```python
from build123d import *

# Parameters (mm, degrees)
ESTRUSIONE_ESTRUSIONE1_DEPTH           = 20
FORO_SVASATO_PER_VITE_M4_1_D           = 4.5
FORO_SVASATO_PER_VITE_M4_1_DEPTH       = 30
FORO_SVASATO_PER_VITE_M4_1_CSINK_D     = 9.4
FORO_SVASATO_PER_VITE_M4_1_CSINK_ANGLE = 90
FORO_SVASATO_PER_VITE_M4_1_TIP         = 1.351936393


with BuildPart() as part:
    # Schizzo1 → Estrusione-Estrusione1 (new body)
    with BuildSketch(Plane.XY):
        with BuildLine():
            Line((-88.074783565, -50.85), (-79.414529527, -45.85))
            ThreePointArc((-79.414529527, -45.85), (-79.414529527, 45.85), (0, 91.7))
            Line((0, 91.7), (0, 101.7))
            ThreePointArc((0, 101.7), (-88.074783565, 50.85), (-88.074783565, -50.85))
        make_face()
        with BuildLine():
            Line((-77.906719865, -65.371499905), (-70.246275434, -58.943623808))
            ThreePointArc((-70.246275434, -58.943623808), (-75.116242461, -52.596959213), (-79.414529527, -45.85))
            Line((-79.414529527, -45.85), (-88.074783565, -50.85))
            ThreePointArc((-88.074783565, -50.85), (-83.307762904, -58.332723577), (-77.906719865, -65.371499905))
        make_face()
    extrude(amount=ESTRUSIONE_ESTRUSIONE1_DEPTH)

    # Foro svasato per Vite M4-1
    with Locations(Plane(origin=(-88.074783565, -50.85, 10), x_dir=(0.5, -0.866025403784, 0), z_dir=(-0.866025403784, -0.5, 0))):
        with Locations((0, 0)):
            CounterSinkHole(FORO_SVASATO_PER_VITE_M4_1_D / 2, FORO_SVASATO_PER_VITE_M4_1_CSINK_D / 2, depth=FORO_SVASATO_PER_VITE_M4_1_DEPTH, counter_sink_angle=FORO_SVASATO_PER_VITE_M4_1_CSINK_ANGLE)
            with Locations((0, 0, -(FORO_SVASATO_PER_VITE_M4_1_DEPTH + FORO_SVASATO_PER_VITE_M4_1_TIP / 2))):  # 118° drill point
                Cone(0, FORO_SVASATO_PER_VITE_M4_1_D / 2, FORO_SVASATO_PER_VITE_M4_1_TIP, mode=Mode.SUBTRACT)


solid = part.part
```
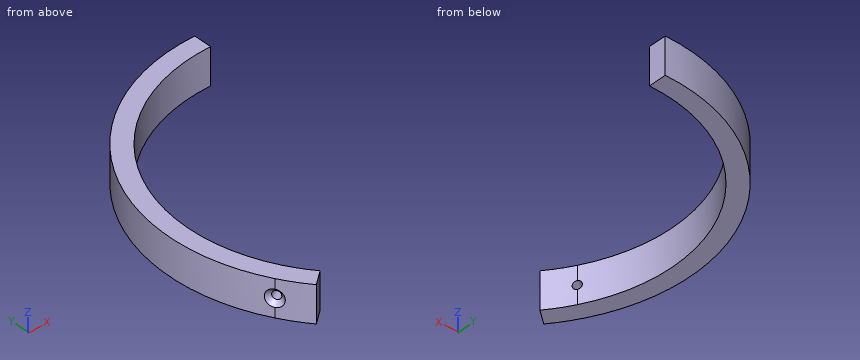
Geometry check sheet. Reference: the model listing, model coordinates, mm. Round coordinates to 2 decimals unless told otherwise and drop trailing zeros. Write each loop counter-clockwise with the first axis right and the second up, starting at its lowest first coordinate (ties: lowest second). Pieces come first, ordered by that corner, then holes. Notation, with made-up numbers: (40, -30) -> (64, -30) arc R23 cw to (64, 0) -> close; hole circle Ø8 at (68.25, -18.5). An arc over 180 degrees is marked (long way). Put each result on its own line as item: value.
1) Depth check by flat-ended pin: P1, Ø4, axis at y = 13, z = 4, coming from the -X side; P2, Ø3, axis at y = -26, z = 2.5, coming from the +X side; P3, Ø1, axis at x = -88, z = 11.5, coming from the -Y side. Enter the tip coordinate at first touch or a pass-through.
Recorded:
P1: stops at x = -101.1
P2: stops at x = -87.48
P3: stops at y = -48.02
2) Cross-section at B-B, the plane x = -29.5. Enter the section's corners in (y, z).
Recorded:
outline: (86.83, 0) -> (97.33, 0) -> (97.33, 20) -> (86.83, 20) -> close
3) Thickness scan on probe 1 along Y at (x, z) = (-83.5, 2.75); probe 2 along Y at (x, z) = (-83, 2.75); probe 3 along X at (y, z) = (-56, 9.5). Record the ranges inside material, lowest first. Write a range as from..to.
Recorded:
probe 1: y = -58.06..-37.9, 37.9..58.06
probe 2: y = -58.77..-38.99, 38.99..58.77
probe 3: x = -84.89..-72.61
4) Cross-section at C-C, the plane y = 19.5. Enter the section's corners in (x, z).
Recorded:
outline: (-99.81, 0) -> (-89.6, 0) -> (-89.6, 20) -> (-99.81, 20) -> close
5) Cross-section at A-A, the plane z = 17.5. Enter the section's corners in (x, y).
Recorded:
outline: (-77.91, -65.37) -> (-70.25, -58.94) arc R91.7 cw to (0, 91.7) -> (0, 101.7) arc R101.7 ccw to start
